Model file for the job. Use its own axes, mm. Coordinates: 2 decimals unless noted, no trailing zeros. Loops run counter-clockwise (first coordinate to the right, second up) from the corner with the lowest first, then second, coordinate; pieces in that order, holes last. Notation, with made-up numbers: M 24.5,1 L 36.5,1 A9 cw 36.5,6 Z; hole C 46,-26.75 d3. An arc over 180 degrees is marked long. Write item = value, one per line. Start each with the question number.
from build123d import *

# Parameters (mm, degrees)
SKETCH1_W           = 465
SKETCH1_H           = 90
SKETCH1_R           = 2.55
BOSS_EXTRUDE1_DEPTH = 2.2479
CUT_EXTRUDE1_REACH  = 6.496
SKETCH2_R           = 1.6
SKETCH2_W           = 58.8
SKETCH2_H           = 20


with BuildPart() as part:
    # Sketch1 → Boss-Extrude1 (new body, symmetric)
    with BuildSketch(Plane.XY):
        Rectangle(SKETCH1_W, SKETCH1_H)
        with Locations((-222.5, 35)):
            Circle(SKETCH1_R, mode=Mode.SUBTRACT)
        with Locations((-222.5, -35)):
            Circle(SKETCH1_R, mode=Mode.SUBTRACT)
        with Locations((0, 35)):
            Circle(SKETCH1_R, mode=Mode.SUBTRACT)
        with Locations((-114.975, 35)):
            Circle(SKETCH1_R, mode=Mode.SUBTRACT)
        with Locations((222.5, -35)):
            Circle(SKETCH1_R, mode=Mode.SUBTRACT)
        with Locations((222.5, 35)):
            Circle(SKETCH1_R, mode=Mode.SUBTRACT)
        with Locations((114.975, 35)):
            Circle(SKETCH1_R, mode=Mode.SUBTRACT)
    extrude(amount=BOSS_EXTRUDE1_DEPTH, both=True)

    # Sketch2 → Cut-Extrude1 (cut, up to next)
    with BuildSketch(Plane.XY.offset(2.2479), mode=Mode.PRIVATE) as cut_extrude1_sk1:
        with Locations((-136.600006438, -5)):
            Circle(SKETCH2_R)
    cut_extrude1_tool1 = extrude(cut_extrude1_sk1.sketch, amount=-CUT_EXTRUDE1_REACH, mode=Mode.PRIVATE) & part.part
    add(cut_extrude1_tool1.solids().sort_by_distance((-136.600006, -5, 2.2479))[0], mode=Mode.SUBTRACT)
    # Sketch2 → Cut-Extrude1 (cut, up to next)
    with BuildSketch(Plane.XY.offset(2.2479), mode=Mode.PRIVATE) as cut_extrude1_sk2:
        with Locations((-168.600006438, -5)):
            Circle(SKETCH2_R)
    cut_extrude1_tool2 = extrude(cut_extrude1_sk2.sketch, amount=-CUT_EXTRUDE1_REACH, mode=Mode.PRIVATE) & part.part
    add(cut_extrude1_tool2.solids().sort_by_distance((-168.600006, -5, 2.2479))[0], mode=Mode.SUBTRACT)
    # Sketch2 → Cut-Extrude1 (cut, up to next)
    with BuildSketch(Plane.XY.offset(2.2479), mode=Mode.PRIVATE) as cut_extrude1_sk3:
        with Locations((-168.600006438, -37)):
            Circle(SKETCH2_R)
    cut_extrude1_tool3 = extrude(cut_extrude1_sk3.sketch, amount=-CUT_EXTRUDE1_REACH, mode=Mode.PRIVATE) & part.part
    add(cut_extrude1_tool3.solids().sort_by_distance((-168.600006, -37, 2.2479))[0], mode=Mode.SUBTRACT)
    # Sketch2 → Cut-Extrude1 (cut, up to next)
    with BuildSketch(Plane.XY.offset(2.2479), mode=Mode.PRIVATE) as cut_extrude1_sk4:
        with Locations((-136.600006438, -37)):
            Circle(SKETCH2_R)
    cut_extrude1_tool4 = extrude(cut_extrude1_sk4.sketch, amount=-CUT_EXTRUDE1_REACH, mode=Mode.PRIVATE) & part.part
    add(cut_extrude1_tool4.solids().sort_by_distance((-136.600006, -37, 2.2479))[0], mode=Mode.SUBTRACT)
    # Sketch2 → Cut-Extrude1 (cut, up to next)
    with BuildSketch(Plane.XY.offset(2.2479), mode=Mode.PRIVATE) as cut_extrude1_sk5:
        Polygon((-108.747160909, 16), (-72.422339974, 16), (-72.422339974, 23), (-50.542339974, 23), (-50.542339974, -6.43), (-108.747160909, -6.43), align=None)
    cut_extrude1_tool5 = extrude(cut_extrude1_sk5.sketch, amount=-CUT_EXTRUDE1_REACH, mode=Mode.PRIVATE) & part.part
    add(cut_extrude1_tool5.solids().sort_by_distance((-77.737733, 6.330046, 2.2479))[0], mode=Mode.SUBTRACT)
    # Sketch2 → Cut-Extrude1 (cut, up to next)
    with BuildSketch(Plane.XY.offset(2.2479), mode=Mode.PRIVATE) as cut_extrude1_sk6:
        with Locations((-152.600006438, 13)):
            Rectangle(SKETCH2_W, SKETCH2_H)
    cut_extrude1_tool6 = extrude(cut_extrude1_sk6.sketch, amount=-CUT_EXTRUDE1_REACH, mode=Mode.PRIVATE) & part.part
    add(cut_extrude1_tool6.solids().sort_by_distance((-152.600006, 13, 2.2479))[0], mode=Mode.SUBTRACT)
    # Sketch2 → Cut-Extrude1 (cut, up to next)
    with BuildSketch(Plane.XY.offset(2.2479), mode=Mode.PRIVATE) as cut_extrude1_sk7:
        with BuildLine():
            ThreePointArc((-163.627957833, -36.472048604), (-152.600006438, -40), (-141.572055042, -36.472048604))
            ThreePointArc((-141.572055042, -36.472048604), (-140.135540343, -33.464466094), (-137.127957833, -32.027951396))
            ThreePointArc((-137.127957833, -32.027951396), (-133.600006437, -21), (-137.127957833, -9.972048604))
            ThreePointArc((-137.127957833, -9.972048604), (-140.135540343, -8.535533906), (-141.572055042, -5.527951396))
            ThreePointArc((-141.572055042, -5.527951396), (-152.600006438, -2), (-163.627957833, -5.527951396))
            ThreePointArc((-163.627957833, -5.527951396), (-165.064472532, -8.535533906), (-168.072055042, -9.972048604))
            ThreePointArc((-168.072055042, -9.972048604), (-171.600006437, -21), (-168.072055042, -32.027951396))
            ThreePointArc((-168.072055042, -32.027951396), (-165.064472532, -33.464466094), (-163.627957833, -36.472048604))
        make_face()
    cut_extrude1_tool7 = extrude(cut_extrude1_sk7.sketch, amount=-CUT_EXTRUDE1_REACH, mode=Mode.PRIVATE) & part.part
    add(cut_extrude1_tool7.solids().sort_by_distance((-152.600006, -21, 2.2479))[0], mode=Mode.SUBTRACT)


solid = part.part
Item 1: Cut at B-B (z = 0.95). Give the number of separate pieces and of enclosed holes in the cut face, plus the area to 3 significant figures.
Item 2: Probe L1, parallel to Y at x = -222.5, z = 0.7; L2, parallel to Y at x = -51, z = -2; L3, parallel to Y at x = -73, z = 0.45. List the from-to ranges inside material, lowest first.
Item 3: Cut at A-A (x = -101). Give the cut face in (y, z), plus the area to 3 significant figures.
Reported:
q1.separate_pieces = 1
q1.enclosed_holes = 14
q1.area = 37,900 mm^2
q2.L1 = -45 to -37.55, -32.45 to 32.45, 37.55 to 45
q2.L2 = -45 to -6.43, 23 to 45
q2.L3 = -45 to -6.43, 16 to 45
q3.outline = M -45,-2.25 L -6.43,-2.25 L -6.43,2.25 L -45,2.25 Z; M 16,-2.25 L 45,-2.25 L 45,2.25 L 16,2.25 Z
q3.area = 304 mm^2
